```python
from build123d import *

# Parameters (mm, degrees)
EXTRUDE_1_DEPTH             = 89
CUT_EXTRUDE_1_DEPTH         = 77.5
SKETCH_4_R                  = 13
CUT_EXTRUDE_2_DEPTH         = 530.874608663
PATTERN_LINEAR_1_COUNT      = 4
PATTERN_LINEAR_1_PITCH      = 80
PATTERN_LINEAR_1_COUNT_DIR2 = 3
PATTERN_LINEAR_1_PITCH_DIR2 = 80
SKETCH_5_R                  = 13
CUT_EXTRUDE_3_DEPTH         = 530.874608663
PATTERN_LINEAR_2_COUNT      = 4
PATTERN_LINEAR_2_PITCH      = 80
PATTERN_LINEAR_2_COUNT_DIR2 = 3
PATTERN_LINEAR_2_PITCH_DIR2 = 80


with BuildPart() as part:
    # 草图2 → 凸台-拉伸1 (new body)
    with BuildSketch(Plane.XY):
        Polygon((15.153077165, 150), (445, 150), (445, -150), (-15.153077165, -150), (-466.009174215, -57.969384567), (-406.009174215, 235.969384567), align=None)
    extrude(amount=EXTRUDE_1_DEPTH)

    # 草图3 → 切除-拉伸1 (cut)
    with BuildSketch(Plane.XY.offset(89)):
        Polygon((-408.709174215, 222.742139956), (13.78930022, 136.5), (445, 136.5), (445, -136.5), (-13.78930022, -136.5), (-463.309174215, -44.742139956), align=None)
    extrude(amount=-CUT_EXTRUDE_1_DEPTH, mode=Mode.SUBTRACT)

    # 草图4 → 切除-拉伸2 (cut, through all)
    with BuildSketch(Plane(origin=(0, 0, 0), x_dir=(-1, 0, 0), z_dir=(0, 0, -1))):
        with Locations((-390, 80)):
            Circle(SKETCH_4_R)
    cut_extrude_2 = extrude(amount=-CUT_EXTRUDE_2_DEPTH, mode=Mode.SUBTRACT)

    # 阵列(线性)1: Cut-Extrude 2 4 × 3
    with Locations(*[(-i * PATTERN_LINEAR_1_PITCH, -j * PATTERN_LINEAR_1_PITCH_DIR2, 0) for i in range(PATTERN_LINEAR_1_COUNT) for j in range(PATTERN_LINEAR_1_COUNT_DIR2) if (i, j) != (0, 0)]):
        add(cut_extrude_2, mode=Mode.SUBTRACT)

    # 草图5 → 切除-拉伸3 (cut, through all)
    with BuildSketch(Plane(origin=(0, 0, 0), x_dir=(-1, 0, 0), z_dir=(0, 0, -1))):
        with Locations((366.120399874, 156.383671769)):
            Circle(SKETCH_5_R)
    cut_extrude_3 = extrude(amount=-CUT_EXTRUDE_3_DEPTH, mode=Mode.SUBTRACT)

    # 阵列(线性)2: Cut-Extrude 3 4 × 3
    with Locations(*[Vector(0.9797958971132713, -0.2000000000000002, 0) * (i * PATTERN_LINEAR_2_PITCH) + Vector(-0.20000000000000018, -0.9797958971132713, 0) * (j * PATTERN_LINEAR_2_PITCH_DIR2) for i in range(PATTERN_LINEAR_2_COUNT) for j in range(PATTERN_LINEAR_2_COUNT_DIR2) if (i, j) != (0, 0)]):
        add(cut_extrude_3, mode=Mode.SUBTRACT)


solid = part.part
```
Geometry check sheet. Reference: the model listing, model coordinates, mm. A direction names the side the tool comes from. Round coordinates to 2 decimals unless told otherwise and drop trailing zeros. Order: outer loops, then holes, each group sorted by start corner. A loop starts at its lowest first (then second) coordinate and runs counter-clockwise, first axis right, second up. Notation, with made-up numbers: M 81,70 L 114,70 A35 cw 114,107 Z; hole C 8.5,29 d5. An arc over 180 degrees is marked long. Answer as CSV lines item,"result".
1) Sectioned sample at C-C on x = 284.5. Record the cut outline in (y, z).
Entries:
outline,"M -150,0 L 150,0 L 150,89 L 136.5,89 L 136.5,11.5 L -136.5,11.5 L -136.5,89 L -150,89 Z"
2) Sectioned sample at B-B on z = 21.5. Record the cut outline in (x, y).
Entries:
outline,"M -466.01,-57.97 L -15.15,-150 L 445,-150 L 445,-136.5 L -13.79,-136.5 L -463.31,-44.74 Z; M -408.71,222.74 L 13.79,136.5 L 445,136.5 L 445,150 L 15.15,150 L -406.01,235.97 Z"
3) Mould release check, pull along Y, two halves, no side actions. Record for faces 1 (the face through (242.987, 80.572, 5.67)), 2 (the face through (445, 1, 11)), 3 (the face through (-436.15, 88.31, 11.33)): +Y half, -Y half, draft (parallel to the pull), parting line (faces both ways), or undercut.
Entries:
face 1,"undercut"
face 2,"draft"
face 3,"+Y half"
4) Gauge pin test, flat ends, axial feed: pin 1 Ø15.5 at (x, y) = (-162.97, -48.38) entering from -Z; pin 2 Ø8 at (x, z) = (-150.5, 75.5) entering from +Y; pin 3 Ø1 at (x, z) = (-100, 52) entering from +Y; pin 4 Ø2 at (x, y) = (-30, 108.5) entering from +Z. Record the tip position at first contact, or that the pin passes through.
Entries:
pin 1,"through"
pin 2,"y = 184.63"
pin 3,"y = 173.61"
pin 4,"z = 11.5"
5) Sectioned sample at D-D on y = -80. Record the cut outline in (x, z), and give its area (3 significant figures).
Entries:
outline,"M -358.08,0 L 137,0 L 137,11.5 L -290.58,11.5 L -290.58,89 L -358.08,89 Z; M 163,0 L 217,0 L 217,11.5 L 163,11.5 Z; M 243,0 L 297,0 L 297,11.5 L 243,11.5 Z; M 323,0 L 377,0 L 377,11.5 L 323,11.5 Z; M 403,0 L 445,0 L 445,11.5 L 403,11.5 Z"
area,"13,300 mm2"
6) Thickness scan on probe 1 along Y at (x, z) = (150, 5); probe 2 along Y at (x, z) = (283, 18.5); probe 3 along Z at (x, y) = (-116, 94). Record the ranges inside material, lowest first. Write a range as [from, to].
Entries:
probe 1,"[-150, -93], [-67, -13], [13, 67], [93, 150]"
probe 2,"[-150, -136.5], [136.5, 150]"
probe 3,"[0, 11.5]"
7) Sectioned sample at A-A on x = 150. Record the cut outline in (y, z).
Entries:
outline,"M -150,0 L -93,0 L -93,11.5 L -136.5,11.5 L -136.5,89 L -150,89 Z; M -67,0 L -13,0 L -13,11.5 L -67,11.5 Z; M 13,0 L 67,0 L 67,11.5 L 13,11.5 Z; M 93,0 L 150,0 L 150,89 L 136.5,89 L 136.5,11.5 L 93,11.5 Z"
8) Tool access check on faces 4 (the face through (-200.417, 180.225, 50.793)), 5 (the face through (-235.403, -91.263, 50.793)), 6 (the face through (226, 136.5, 51)). Record the directions out of +Z, -Z, +X, -X, +Y, -Y that give a thin tool (end or side, any length) a straight path to the whole face; none if there is none.
Entries:
face 4,"+Z, -X"
face 5,"+Z, +X"
face 6,"+Z, +X, -X"
